Could you check a few things on this model? Use its own coordinates, in mm. Coordinates: 2 decimals unless noted, no trailing zeros. Order: outer loops, then holes, each group sorted by start corner. A loop starts at its lowest first (then second) coordinate and runs counter-clockwise, first axis right, second up. Notation, with made-up numbers: (0, -5) -> (8, -5) arc R28 cw to (8, 26) -> close; hole circle Ø8 at (53.25, 84.5). An arc over 180 degrees is marked (long way). Use a Markdown table: item, result. Add a question column.
1) Will this pin go through, and if not, where does the flat tip stop? pin 1 Ø2 at (x, z) = (2, 0) entering from +Y.
2) If we section it at C-C (y = -5): Write out the boundary of the cut face in (x, z) (3 decimals), plus the area to 3 significant figures.
3) If we section it at A-A (z = -0.5): Write out the boundary of the cut face in (x, y) (3 decimals).
4) If we section it at B-B (x = 2.75): Write out the boundary of the cut face in (y, z) (3 decimals), plus the area to 3 significant figures.
5) If I drill on L1, parallel to Y at x = 0.5, z = -2; L2, parallel to Y at x = 2.5, z = 1.5, over which ranges is the centre line in solid material (lowest first)? Write a range as [from, to].
```python
from build123d import *

# Parameters (mm, degrees)
F0_W     = 6.35
F0_H     = 6.35
F1_DEPTH = 50.8
F6_DEPTH = 25.4
F8_DEPTH = 25.4


with BuildPart() as f1:
    # F0 (on Front) → F1 (new body)
    with BuildSketch(Plane.XZ):
        Rectangle(F0_W, F0_H)
    extrude(amount=F1_DEPTH)

    # F5: sweep along a path in F4
    with BuildLine(Plane.XY.offset(3.175)) as f5_path:
        Line((0, 0), (-7.3544457124, -12.7382736354))
    # F3 (on face) → F5 (sweep, cut)
    with BuildSketch(Plane(origin=(0, 0, 0), x_dir=(-1, 0, 0), z_dir=(0, 1, 0))):
        Polygon((0, -3.175), (0, 3.175), (-1.3497341666, -3.175), align=None)
    sweep(path=f5_path.line, mode=Mode.SUBTRACT)

    # F2 (on face) → F6 (cut)
    with BuildSketch(Plane.XY.offset(3.175)):
        Polygon((-3.175, -5.499261314), (0, 0), (-3.175, 0), align=None)
    extrude(amount=-F6_DEPTH, mode=Mode.SUBTRACT)

    # F7: sweep along a path in F4
    with BuildLine(Plane.XY.offset(3.175)) as f7_path:
        Line((0, 0), (31.0128101016, -21.7154034142))
    # F3 (on face) → F7 (sweep, cut)
    with BuildSketch(Plane(origin=(0, 0, 0), x_dir=(-1, 0, 0), z_dir=(0, 1, 0))):
        Polygon((1.3497341666, -3.175), (0, 3.175), (0, -3.175), align=None)
    sweep(path=f7_path.line, mode=Mode.SUBTRACT)

    # F4 (on face) → F8 (cut)
    with BuildSketch(Plane.XY.offset(3.175)):
        Polygon((3.175, 0), (0, 0), (3.175, -2.2231589338), align=None)
    extrude(amount=-F8_DEPTH, mode=Mode.SUBTRACT)


solid = f1.part
```
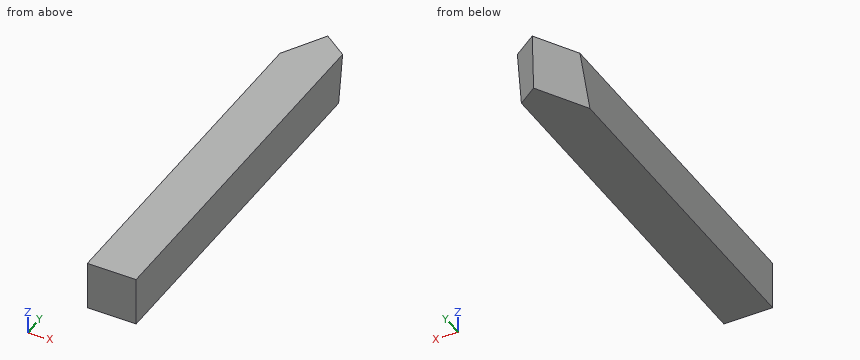
Answer sheet:
| question | item | result |
|---|---|---|
| 1 | pin 1 | y = -1.16 |
| 2 | outline | (-2.887, 3.175) -> (-1.537, -3.175) -> (3.175, -3.175) -> (3.175, 3.175) -> close |
| 2 | area | 34.2 mm2 |
| 3 | outline | (-3.175, -50.8) -> (3.175, -50.8) -> (3.175, -2.77) -> (0.331, -0.779) -> (-3.175, -6.852) -> close |
| 4 | outline | (-50.8, -3.175) -> (-2.871, -3.175) -> (-1.926, 3.175) -> (-50.8, 3.175) -> close |
| 4 | area | 307 mm2 |
| 5 | L1 | [-50.8, -1.12] |
| 5 | L2 | [-50.8, -2] |
